Design review of the part built by this model. Coordinates are the model's own, in mm. A direction names the side the tool comes from. Give positions to 0.01 mm unless a question says otherwise; leave off trailing zeros. Loops run counter-clockwise (first coordinate to the right, second up) from the corner with the lowest first, then second, coordinate; pieces in that order, holes last. Notation, with made-up numbers: (-10.75, 3.25) -> (38.25, 3.25) arc R6 ccw to (38.25, 7.25) -> close; hole circle Ø8 at (30.25, 80). An arc over 180 degrees is marked (long way). Use CSV: the item, a comma, the result in double quotes. Start each with the question number.
Item 1: Clearance check with flat-ended pins moving along their axes: pin 1 (1 mm diameter, centred on x = -5, z = 12.5, fed in from +Y); pin 2 (3 mm diameter, centred on y = 28, z = 12.5, fed in from -X); pin 3 (2 mm diameter, centred on x = -1.5, y = 4, fed in from -Z). State where each tip first meets the part, or that it passes through.
Item 2: Wall thickness on line 1 along X through (y, z) = (31.35, 0); line 2 along Y through (x, z) = (0.5, -13): over which ranges is each line inside the solid? List them lowest first. Write a range as from..to.
Item 3: We need section A-A (z = 0). State the section outline as (x, y) points.
Item 4: We need section C-C (y = 20). State the section outline as (x, z) points, plus the area to 3 significant figures.
Item 5: We need section B-B (x = 0). State the section outline as (y, z) points.
Item 6: We need section D-D (y = 42.5). State the section outline as (x, z) points.
Item 7: For faces 4 (the face through (13.887, 14.79, 10.648)), 5 (the face through (-0.596, -0.246, 2.685)), 6 (the face through (-0.54, 43.31, -2.44)), list the 3-axis set-ups (+Z, -Z, +X, -X, +Y, -Y) from which the entire face can be reached by the end or side of a thin tool; tool diameter is ignored.
Item 8: The part is to be moulded in two halves that separate along Z. For faces 1 (the face through (-0.54, -0.99, 2.44)), 2 (the face through (0, -2, 0)), 3 (the face through (-0.59, 31.48, 4.46)), say which applies: +Z half, -Z half, draft (parallel to the pull), parting line (faces both ways), or undercut.
Autodesk Inventor part; units mm, degrees
ref_plane "YZ Plane" through (0, 0, 0) normal (1, 0, 0) x (0, 1, 0)
ref_plane "XZ Plane" through (0, 0, 0) normal (0, 1, 0) x (-1, 0, 0)
ref_plane "XY Plane" through (0, 0, 0) normal (0, 0, 1) x (1, 0, 0)
sketch "Sketch1" plane through (0, 0, 0) normal (0, 1, 0) x (-1, 0, 0)
  circle A0 centre (0, 0) radius 17.5
  dimension "d0" = 35
extrude "Extrusion1" add sketch "Sketch1" along normal blind 30
sketch "Sketch2" plane through (0, 0, 0) normal (0, -1, 0) x (1, 0, 0)
  circle A0 centre (0, 0) radius 2.5
  dimension "d3" = 5
extrude "Extrusion2" add sketch "Sketch2" along normal blind 2
sketch "Sketch3" plane through (0, 30, 0) normal (0, 1, 0) x (1, 0, 0)
  circle A0 centre (0, 0) radius 2.5
  dimension "d6" = 5
extrude "Extrusion3" add sketch "Sketch3" along normal blind 27
sketch "Sketch4" plane through (0, 30, 0) normal (0, 1, 0) x (1, 0, 0)
  circle A0 centre (0, 0) radius 4.5
  circle A1 centre (0, 0) radius 2.75
  dimension "d9" = 9
  dimension "d12" = 5.5
extrude "Extrusion5" add sketch "Sketch4" along normal blind 3
sketch "Sketch5" plane through (0, 0, 0) normal (0, -1, 0) x (1, 0, 0)
  circle A0 centre (0, 0) radius 2.75
  circle A1 centre (0, 0) radius 4.5
  dimension "d15" = 5.5
  dimension "d16" = 9
extrude "Extrusion6" add sketch "Sketch5" along normal blind 0.5
Results found:
1,pin 1,"y = 30"
1,pin 2,"x = -13.61"
1,pin 3,"z = -17.49"
2,line 1,"-4.5..-2.75, -2.5..2.5, 2.75..4.5"
2,line 2,"0..30"
3,outline,"(-17.5, 0) -> (-4.5, 0) -> (-4.5, -0.5) -> (-2.75, -0.5) -> (-2.75, 0) -> (-2.5, 0) -> (-2.5, -2) -> (2.5, -2) -> (2.5, 0) -> (2.75, 0) -> (2.75, -0.5) -> (4.5, -0.5) -> (4.5, 0) -> (17.5, 0) -> (17.5, 30) -> (4.5, 30) -> (4.5, 33) -> (2.75, 33) -> (2.75, 30) -> (2.5, 30) -> (2.5, 57) -> (-2.5, 57) -> (-2.5, 30) -> (-2.75, 30) -> (-2.75, 33) -> (-4.5, 33) -> (-4.5, 30) -> (-17.5, 30) -> close"
4,outline,"circle Ø35 at (0, 0)"
4,area,"962 mm²"
5,outline,"(-2, -2.5) -> (0, -2.5) -> (0, -2.75) -> (-0.5, -2.75) -> (-0.5, -4.5) -> (0, -4.5) -> (0, -17.5) -> (30, -17.5) -> (30, -4.5) -> (33, -4.5) -> (33, -2.75) -> (30, -2.75) -> (30, -2.5) -> (57, -2.5) -> (57, 2.5) -> (30, 2.5) -> (30, 2.75) -> (33, 2.75) -> (33, 4.5) -> (30, 4.5) -> (30, 17.5) -> (0, 17.5) -> (0, 4.5) -> (-0.5, 4.5) -> (-0.5, 2.75) -> (0, 2.75) -> (0, 2.5) -> (-2, 2.5) -> close"
6,outline,"circle Ø5 at (0, 0)"
7,face 4,"+Y, -Y"
7,face 5,"-Y"
7,face 6,"+Y"
8,face 1,"undercut"
8,face 2,"draft"
8,face 3,"parting line"
